Can you work these out from the drawing? Everything is in mm from the part's minimum corner. Coordinates: 2 decimals unless noted, no trailing zeros. Order: outer loops, then holes, each group sorted by start corner. A loop starts at its lowest first (then second) coordinate and runs counter-clockwise, first axis right, second up. Notation, with made-up numbers: (43, 55) - (63, 55) arc R28 ccw to (63, 74) - close; hole circle Ø8 at (-27, 46.5). An arc over 180 degrees is marked (long way). One line per item, written item: value.
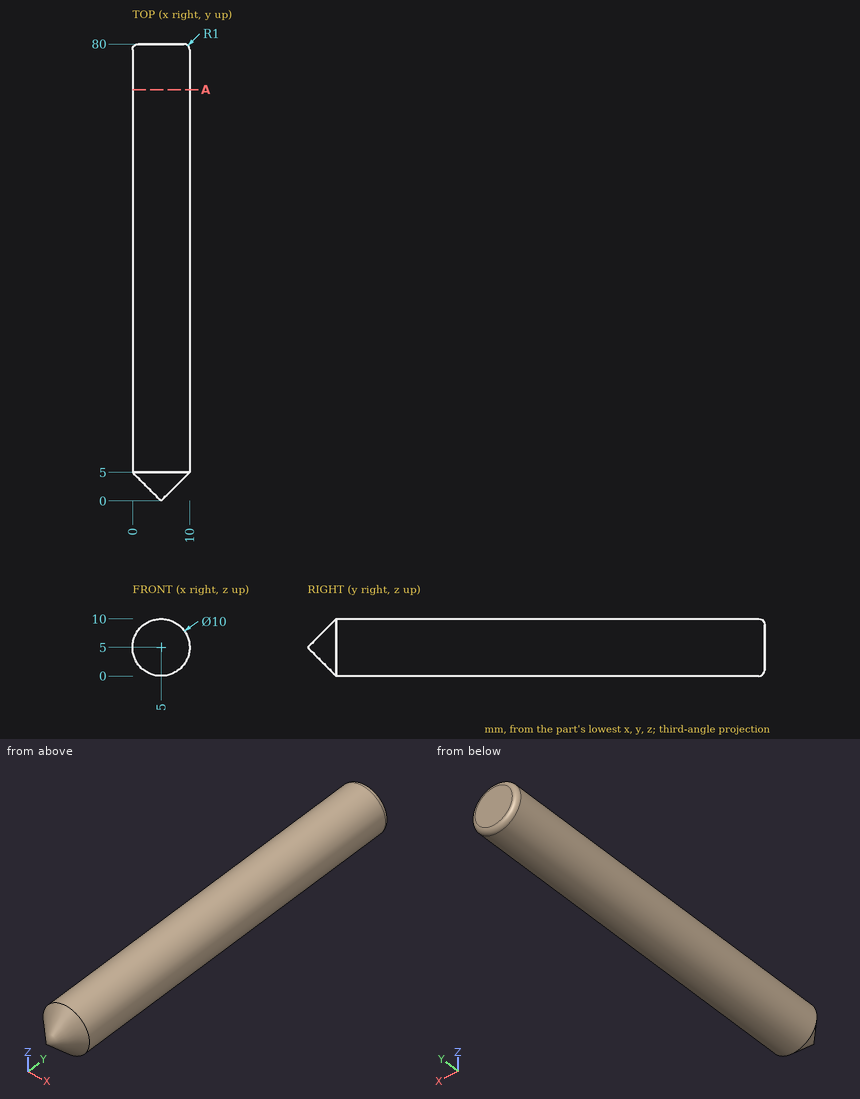
Item 1: I want a section at A-A on y = 72. Please give me the cut outline in (x, z), then the cut area to 3 significant figures.
Conclusion:
outline: circle Ø10 at (5, 5)
area: 78.5 mm²
Item 2: I'm going to push flat-ended pins straight in: pin 1 Ø3 at (x, z) = (2, 7.5) entering from -Y; pin 2 Ø5 at (y, z) = (12, 5.5) entering from +X; pin 3 Ø2 at (x, y) = (7, 16) entering from -Z; pin 4 Ø5 at (x, z) = (3.5, 8.5) entering from -Y. Where does each tip first touch, or does it pass through?
Conclusion:
pin 1: y = 2.41
pin 2: x = 10
pin 3: z = 0.1
pin 4: y = 1.31
Item 3: If I drill on probe 1 along Z at (x, y) = (8, 32); probe 2 along Z at (x, y) = (7, 24); probe 3 along Y at (x, z) = (6.5, 8.5), over which ranges is the centre line in solid material (lowest first)?
Conclusion:
probe 1: 1 to 9
probe 2: 0.42 to 9.58
probe 3: 3.81 to 80
